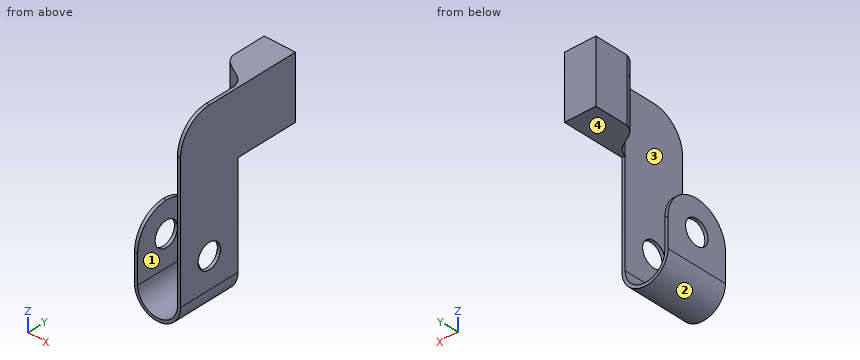
```python
from build123d import *

# Parameters (mm, degrees)
F1_DEPTH  = 10
F0_W      = 0.5
F0_H      = 10
F2_DEPTH  = 10
F3_DEPTH  = 10
F4_R      = 1.95
F5_DEPTH  = 25
F6_DEPTH  = 25
F7_R      = 4.99999
F4_W      = 10
F4_H      = 10
F8_DEPTH  = 4.5
F10_DEPTH = 25


# Not quite as in the source:
# - a fillet or chamfer is up to 0.001 mm smaller than in the source, because OpenCascade refuses the exact size


with BuildPart() as f1:
    # F0 (on Front) → F1 (new body)
    with BuildSketch(Plane.XZ):
        with BuildLine():
            Line((0.5, 3.675), (0, 3.675))
            ThreePointArc((0, 3.675), (3.675, 0), (7.35, 3.675))
            Line((7.35, 3.675), (7.35, 20))
            Line((7.35, 20), (6.85, 20))
            Line((6.85, 20), (6.85, 3.675))
            ThreePointArc((6.85, 3.675), (3.675, 0.5), (0.5, 3.675))
        make_face()
        Polygon((0, 11.5236516859), (0, 3.675), (0.5, 3.675), (0.5, 13.3078707406), (0, 13.3078707406), align=None)
    extrude(amount=F1_DEPTH)

    # F0 (on Front) → F2 (join)
    with BuildSketch(Plane.XZ):
        with Locations((7.1, 25)):
            Rectangle(F0_W, F0_H)
    extrude(amount=F2_DEPTH)

    # F0 (on Front) → F3 (join)
    with BuildSketch(Plane.XZ):
        with Locations((7.1, 25)):
            Rectangle(F0_W, F0_H)
    extrude(amount=-F3_DEPTH)

    # F4 (on face) → F5 (cut)
    with BuildSketch(Plane(origin=(6.85, 0, 0), x_dir=(0, -1, 0), z_dir=(-1, 0, 0))):
        with Locations((5.0057064388, 8.4952701442)):
            Circle(F4_R)
    extrude(amount=-F5_DEPTH, mode=Mode.SUBTRACT)

    # F4 (on face) → F6 (cut)
    with BuildSketch(Plane(origin=(6.85, 0, 0), x_dir=(0, -1, 0), z_dir=(-1, 0, 0))):
        with Locations((5.0057064388, 8.4952701442)):
            Circle(F4_R)
    extrude(amount=F6_DEPTH, mode=Mode.SUBTRACT)

    # F7 (radius 5 in the source; OpenCascade refuses exactly that, so slightly less here)
    f7_edges = [f1.edges().sort_by_distance(p)[0] for p in [
        (7.1, -10, 30),
        (0.25, -10, 13.307871),
        (0.25, 0, 13.307871),
    ]]
    fillet(f7_edges, radius=F7_R)

    # F4 (on face) → F8 (join)
    with BuildSketch(Plane(origin=(6.85, 0, 0), x_dir=(0, -1, 0), z_dir=(-1, 0, 0))):
        with Locations((-5, 25)):
            Rectangle(F4_W, F4_H)
    extrude(amount=F8_DEPTH)

    # F9 (on face) → F10 (cut)
    with BuildSketch(Plane.XY.offset(30)):
        with BuildLine():
            Line((2.35, 0), (6.85, 0))
            add(Edge.make_bspline(
                [(6.85, 0), (6.6607907806, 0.4988620131), (6.3387521568, 1.6560182736), (2.9528697619, 2.8701009159), (2.4258734683, 4.2211432066), (2.35, 4.5559741557)],
                knots=[0, 0, 0, 0, 0.2515030108, 0.6187434404, 0.8676489933, 0.8676489933, 0.8676489933, 0.8676489933], degree=3))
            Line((2.35, 4.5559741557), (2.35, 0))
        make_face()
    extrude(amount=-F10_DEPTH, mode=Mode.SUBTRACT)


solid = f1.part
```
Design review of the part built by this model. Coordinates are the model's own, in mm. Face numbers are marked on the shaded views. Coordinates: 2 decimals unless noted, no trailing zeros. Order: outer loops, then holes, each group sorted by start corner. A loop starts at its lowest first (then second) coordinate and runs counter-clockwise, first axis right, second up.
1) Take a section at C-C, the plane y = -5.75. Give the boundary of the cut face in (x, z) (3 decimals).
2) Clearance check with flat-ended pins moving along their axes: pin 1 (3 mm diameter, centred on x = 5, y = -7.5, fed in from +Z); pin 2 (4 mm diameter, centred on x = 5.5, y = 4, fed in from -Z); pin 3 (1.6 mm diameter, centred on y = 8.5, z = 27.5, fed in from -X). State where each tip first meets the part, or that it passes through.
3) Take a section at B-B, the plane y = -8. Give the boundary of the cut face in (x, z) (3 decimals), and give its area (3 significant figures).
4) Take a section at D-D, the plane x = 2. Give the boundary of the cut face in (y, z).
5) Take a section at A-A, the plane z = 5.5. Give the boundary of the cut face in (x, y), and give its area (3 significant figures).
6) Mouldability with a two-part tool opening along X and no side actions: class the marked faces 1, 2, 3 and 4 as +X half, -X half, draft (parallel to the pull), parting line (faces both ways), or undercut.
7) Wall thickness on line 1 along X through (y, z) = (-9, 8); line 2 along Z through (x, y) = (3.75, 5.75); line 3 along X through (y, z) = (-0.75, 14.5): over which ranges is each line inside the solid? List them lowest first.
Returned:
1. outline: (0, 3.675) arc R3.675 ccw to (7.35, 3.675) - (7.35, 6.693) - (6.85, 6.693) - (6.85, 3.675) arc R3.175 cw to (0.5, 3.675) - (0.5, 6.693) - (0, 6.693) - close; (0, 10.298) - (0.5, 10.298) - (0.5, 13.251) - (0, 13.251) - close; (6.85, 10.298) - (7.35, 10.298) - (7.35, 29.943) - (6.85, 29.943) - close
2. pin 1: stops at z = 2.23
2. pin 2: stops at z = 20
2. pin 3: stops at x = 2.35
3. outline: (0, 3.675) arc R3.675 ccw to (7.35, 3.675) - (7.35, 29) - (6.85, 29) - (6.85, 3.675) arc R3.175 cw to (0.5, 3.675) - (0.5, 12.308) - (0, 12.308) - close
3. area: 22.4 mm2
4. outline: (-10, 0.4) - (0, 0.4) - (0, 0.98) - (-10, 0.98) - close
5. outline: (0, -10) - (0.5, -10) - (0.5, 0) - (0, 0) - close; (6.85, -10) - (7.35, -10) - (7.35, 0) - (6.85, 0) - close
5. area: 10.0 mm2
6. face 1: undercut
6. face 2: parting line
6. face 3: undercut
6. face 4: draft
7. line 1: x = 0 to 0.5, 6.85 to 7.35
7. line 2: z = 20 to 30
7. line 3: x = 6.85 to 7.35
